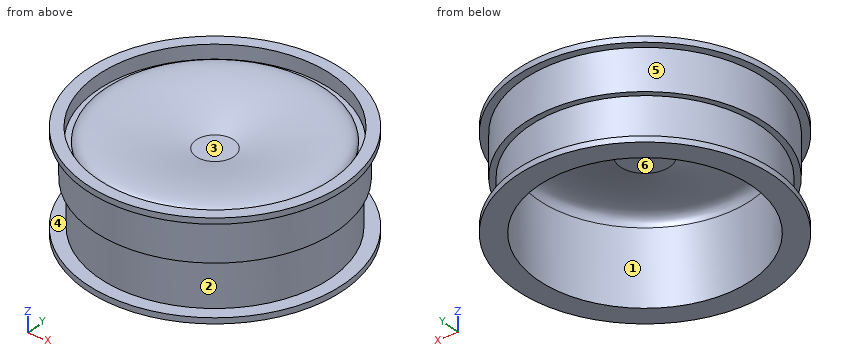
from build123d import *


with BuildPart() as part:
    # Sketch1 → Revolve2 (revolve)
    with BuildSketch(Plane(origin=(0, 0, 0), x_dir=(0, 0, -1), z_dir=(1, 0, 0)), mode=Mode.PRIVATE) as revolve2_sk:
        with BuildLine():
            Line((0, 0), (2.208762887, 0))
            Line((2.208762887, 0), (2.208762887, 7.5))
            add(Edge.make_bspline(
                [(2.208762887, 7.5), (-4.75, 30), (-2, 32.5), (1.246245651, 32.5)],
                knots=[0, 0, 0, 0, 1, 1, 1, 1], degree=3))
            Line((1.246245651, 32.5), (23.996245651, 32.5))
            Line((23.996245651, 32.5), (23.996245651, 39.25))
            Line((23.996245651, 39.25), (22.246245651, 39.25))
            Line((22.246245651, 39.25), (22.246245651, 35.25))
            Line((22.246245651, 35.25), (8.246245651, 35.25))
            Line((8.246245651, 35.25), (8.246245651, 37))
            Line((8.246245651, 37), (-4.253754349, 37))
            Line((-4.253754349, 37), (-4.253754349, 39.25))
            Line((-4.253754349, 39.25), (-6.003754349, 39.25))
            Line((-6.003754349, 39.25), (-6.003754349, 35.75))
            Line((-6.003754349, 35.75), (-1.753754349, 35.75))
            Line((-1.753754349, 35.75), (-1.753754349, 34))
            add(Edge.make_bspline(
                [(0, 5.75), (-7.5, 30), (-4, 34), (-1.753754349, 34)],
                knots=[0, 0, 0, 0, 1, 1, 1, 1], degree=3))
            Line((0, 5.75), (0, 0))
        make_face()
    revolve(revolve2_sk.sketch.rotate(Axis((0, 0, 0), (0, 0, -1)), 90), axis=Axis((0, 0, 0), (0, 0, -1)))


solid = part.part
Verification items for the finished model (mm, model axes). Face numbers are marked on the shaded views. A direction names the side the tool comes from. Coordinates: 2 decimals unless noted, no trailing zeros. Loops run counter-clockwise (first coordinate to the right, second up) from the corner with the lowest first, then second, coordinate; pieces in that order, holes last. Notation, with made-up numbers: (88, 72.25) -> (92, 72.25) arc R19 ccw to (92, 89.25) -> close; hole circle Ø3 at (33, -15). An arc over 180 degrees is marked (long way). Answer as CSV lines item,"result".
1) Tool access check on the marked faces 1, 2 and 3. Record the directions out of +Z, -Z, +X, -X, +Y, -Y that give a thin tool (end or side, any length) a straight path to the whole face; none if there is none.
Found:
face 1,"-Z"
face 2,"none"
face 3,"+Z"
2) Release check for a two-part mould opening along X. For the marked faces 4, 5 and 6 record: +X half, -X half, draft (parallel to the pull), parting line (faces both ways), or undercut.
Found:
face 4,"draft"
face 5,"parting line"
face 6,"undercut"
3) Cross-section at B-B, the plane z = 3.25. Count the separate pieces of the cut face and the enclosed holes in it, then the cut area to 3 significant figures.
Found:
separate pieces,"2"
enclosed holes,"2"
area,"2,760 mm2"
4) Thickness scan on L1, parallel to Y at x = 0, z = -12.25; L2, parallel to Y at x = 0, z = -7.5; L3, parallel to Z at x = 19, y = 30. Record the ranges inside material, lowest first. Write a range as from..to.
Found:
L1,"y = -35.25..-32.5, 32.5..35.25"
L2,"y = -37..-32.5, 32.5..37"
L3,"z = -24..-22.25, -8.25..1.75"
5) Depth check by flat-ended pin: pin 1 (6 mm diameter, centred on x = -14, y = -8.5, fed in from -Z); pin 2 (4 mm diameter, centred on y = -15.5, z = -3, fed in from +X); pin 3 (6 mm diameter, centred on x = 18.5, y = -7, fed in from -Z). Enter the tip coordinate at first touch or a pass-through.
Found:
pin 1,"stops at z = -0.48"
pin 2,"stops at x = 34.45"
pin 3,"stops at z = 0.41"
6) Cross-section at A-A, the plane z = -5. Record the cut outline in (x, y).
Found:
outline,"circle Ø74 at (0, 0); hole circle Ø65 at (0, 0)"
